from build123d import *

# Parameters (mm, degrees)
F0_R     = 1.55
F1_DEPTH = 2.91
F3_DEPTH = 4.8
F4_W     = 130
F4_H     = 88
F4_W_2   = 124
F4_H_2   = 82
F5_DEPTH = 5
F6_DEPTH = 25


with BuildPart() as f1:
    # F0 (on Top) → F1 (new body)
    with BuildSketch(Plane.XY):
        with BuildLine():
            Line((-70.875, -54.61), (70.875, -54.61))
            ThreePointArc((70.875, -54.61), (76.885408, -52.120408), (79.375, -46.11))
            Line((79.375, -46.11), (79.375, 46.11))
            ThreePointArc((79.375, 46.11), (76.885408, 52.120408), (70.875, 54.61))
            Line((70.875, 54.61), (-70.875, 54.61))
            ThreePointArc((-70.875, 54.61), (-76.885408, 52.120408), (-79.375, 46.11))
            Line((-79.375, 46.11), (-79.375, -46.11))
            ThreePointArc((-79.375, -46.11), (-76.885408, -52.120408), (-70.875, -54.61))
        make_face()
        with Locations((71.875, -45.11)):
            Circle(F0_R, mode=Mode.SUBTRACT)
        with Locations((-71.875, 45.11)):
            Circle(F0_R, mode=Mode.SUBTRACT)
    extrude(amount=F1_DEPTH)

    # F2 (on Top) → F3 (join)
    with BuildSketch(Plane.XY):
        Polygon((-62.5, -47.425), (62.5, -47.425), (67.5, -42.425), (67.5, 42.425), (62.5, 47.425), (-62.5, 47.425), (-67.5, 42.425), (-67.5, -42.425), align=None)
    extrude(amount=-F3_DEPTH)

    # F4 (on face) → F5 (cut)
    with BuildSketch(Plane.XY.offset(2.91)):
        Rectangle(F4_W, F4_H)
        Rectangle(F4_W_2, F4_H_2, mode=Mode.SUBTRACT)
        Rectangle(F4_W_2, F4_H_2)
    extrude(amount=-F5_DEPTH, mode=Mode.SUBTRACT)

    # F4 (on face) → F6 (cut)
    with BuildSketch(Plane.XY.offset(2.91)):
        Rectangle(F4_W_2, F4_H_2)
    extrude(amount=-F6_DEPTH, mode=Mode.SUBTRACT)


solid = f1.part
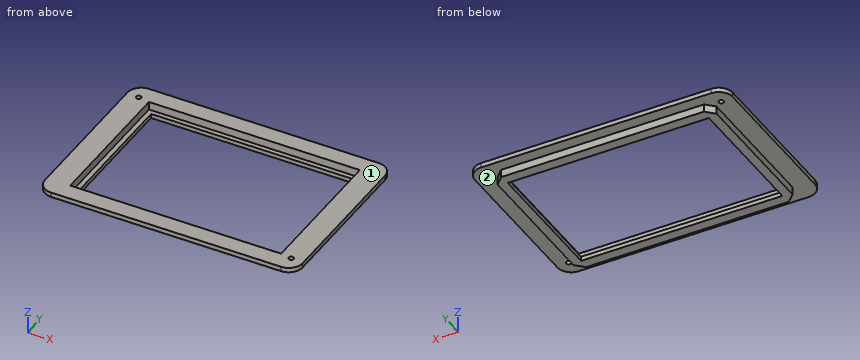
Part model, mm, in its own coordinate system. Face numbers are marked on the shaded views. A direction names the side the tool comes from. Round coordinates to 2 decimals unless told otherwise and drop trailing zeros. Write each loop counter-clockwise with the first axis right and the second up, starting at its lowest first coordinate (ties: lowest second). Pieces come first, ordered by that corner, then holes. Notation, with made-up numbers: M 44.5,-30 L 78.5,-30 A19 ccw 78.5,-1 Z; hole C 6.25,23 d6. An arc over 180 degrees is marked long. Return JSON: item names as keys, results as strings. Group by question number.
(1) Saw through at B-B on y = 26. Write the cut outline in (x, z) (3 decimals), then the cut area to 3 significant figures.
(2) Which spindle directions (+Z, -Z, +X, -X, +Y, -Y) get a long thin tool onto all of the face, cutting with end or side? Do the marked faces 1 and 2. Say none if no direction does.
(3) Drill centre lines: probe 1 along Y at (x, z) = (-46.5, -2) (3 decimals); probe 2 along Y at (x, z) = (-58.5, -3) (3 decimals); probe 3 along X at (y, z) = (22, -4.25). Where is each one in solid material? Low to high.
(4) Pin check, flat tips, straight feed: pin 1 Ø3 at (x, z) = (-26, -3.5) entering from -Y (3 decimals); pin 2 Ø3 at (x, z) = (-7.5, -4) entering from +Y (3 decimals); pin 3 Ø2 at (y, z) = (18, -3) entering from -X; pin 4 Ø2.5 at (x, y) = (71.875, -45.11) entering from -Z. Stop position of each tip, or through.
(5) Saw through at A-A on x = -17. Write the cut outline in (y, z) (3 decimals).
Returned:
{
 "1": {"outline": "M -79.375,0 L -67.5,0 L -67.5,-4.8 L -62,-4.8 L -62,-2.09 L -65,-2.09 L -65,2.91 L -79.375,2.91 Z; M 62,-4.8 L 67.5,-4.8 L 67.5,0 L 79.375,0 L 79.375,2.91 L 65,2.91 L 65,-2.09 L 62,-2.09 Z", "area": "124 mm²"},
 "2": {"face 1": "+Z, +X, -X, +Y, -Y", "face 2": "-Z"},
 "3": {"probe 1": "-47.425 to -44, 44 to 47.425", "probe 2": "-47.425 to -41, 41 to 47.425", "probe 3": "-67.5 to -62, 62 to 67.5"},
 "4": {"pin 1": "y = -47.425", "pin 2": "y = 47.425", "pin 3": "x = -67.5", "pin 4": "through"},
 "5": {"outline": "M -54.61,0 L -47.425,0 L -47.425,-4.8 L -41,-4.8 L -41,-2.09 L -44,-2.09 L -44,2.91 L -54.61,2.91 Z; M 41,-4.8 L 47.425,-4.8 L 47.425,0 L 54.61,0 L 54.61,2.91 L 44,2.91 L 44,-2.09 L 41,-2.09 Z"}
}
